Answer from the drawing. Dimensions are ordinates in mm from the lowest x, y and z of the part. A direction names the side the tool comes from. Coordinates: 2 decimals unless noted, no trailing zeros. Loops run counter-clockwise (first coordinate to the right, second up) from the corner with the lowest first, then second, coordinate; pieces in that order, holes last.
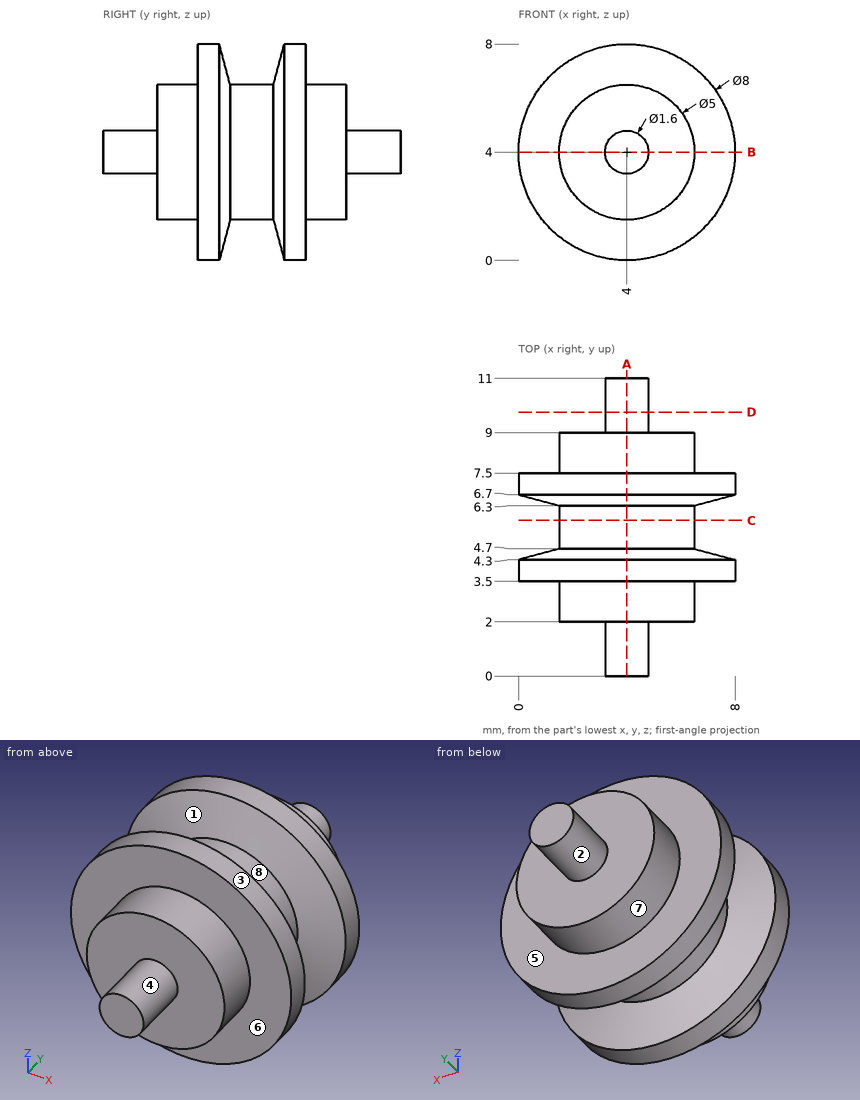
Item 1: Which of the six approach directions +Z, -Z, +X, -X, +Y, -Y give full straight-line access (tool end or side, diameter ignored) to the marked faces 1, 2, 3 and 4?
Numbers:
face 1: none
face 2: +Y
face 3: +Y, -Y
face 4: -Y
Item 2: Find the intervals of material crossed by line 1 along Y through (x, z) = (3, 6); line 2 along Y through (x, z) = (4.75, 6.75); line 3 along Y through (x, z) = (7.5, 2.75), in increasing order.
Numbers:
line 1: y = 2 to 9
line 2: y = 3.5 to 4.61, 6.39 to 7.5
line 3: y = 3.5 to 4.38, 6.62 to 7.5
Item 3: A cutting plane is placed at B-B on z = 4. Determine the outline of the cut face in (x, y).
Numbers:
outline: (0, 3.5) - (1.5, 3.5) - (1.5, 2) - (3.2, 2) - (3.2, 0) - (4.8, 0) - (4.8, 2) - (6.5, 2) - (6.5, 3.5) - (8, 3.5) - (8, 4.3) - (6.5, 4.7) - (6.5, 6.3) - (8, 6.7) - (8, 7.5) - (6.5, 7.5) - (6.5, 9) - (4.8, 9) - (4.8, 11) - (3.2, 11) - (3.2, 9) - (1.5, 9) - (1.5, 7.5) - (0, 7.5) - (0, 6.7) - (1.5, 6.3) - (1.5, 4.7) - (0, 4.3) - close
Item 4: Given pin 1 (2.5 mm diameter, centred on x = 4, z = 3.5, fed in from -Y); pin 2 (2 mm diameter, centred on x = 4, z = 2, fed in from -Y); pin 3 (2 mm diameter, centred on x = 5, y = 3, fed in from +Z); pin 4 (1 mm diameter, centred on x = 5.5, y = 2.5, fed in from +Z), each flat-ended and moving along its own axis, determine where each tip first touches the part or whether it passes through.
Numbers:
pin 1: stops at y = 0
pin 2: stops at y = 2
pin 3: stops at z = 8
pin 4: stops at z = 6.29
Item 5: A cutting plane is placed at C-C on y = 5.75. Determine the outline of the cut face in (x, z), then the cut area to 3 significant figures.
Numbers:
outline: circle Ø5 at (4, 4)
area: 19.6 mm2
Item 6: A cutting plane is placed at D-D on y = 9.75. Determine the outline of the cut face in (x, z), then the cut area to 3 significant figures.
Numbers:
outline: circle Ø1.6 at (4, 4)
area: 2.01 mm2
Item 7: Determine the mould class of the marked faces 5, 6, 7 and 8 for opening direction Y: released by +Y, released by -Y, zero draft, split by the parting line, or undercut.
Numbers:
face 5: released by +Y
face 6: released by -Y
face 7: zero draft
face 8: undercut
Item 8: A cutting plane is placed at A-A on x = 4. Determine the outline of the cut face in (y, z).
Numbers:
outline: (0, 3.2) - (2, 3.2) - (2, 1.5) - (3.5, 1.5) - (3.5, 0) - (4.3, 0) - (4.7, 1.5) - (6.3, 1.5) - (6.7, 0) - (7.5, 0) - (7.5, 1.5) - (9, 1.5) - (9, 3.2) - (11, 3.2) - (11, 4.8) - (9, 4.8) - (9, 6.5) - (7.5, 6.5) - (7.5, 8) - (6.7, 8) - (6.3, 6.5) - (4.7, 6.5) - (4.3, 8) - (3.5, 8) - (3.5, 6.5) - (2, 6.5) - (2, 4.8) - (0, 4.8) - close
